```python
from build123d import *

# Parameters (mm, degrees)
SKETCH1_W           = 42
SKETCH1_H           = 70
SKETCH1_R           = 11.5
SKETCH1_R_2         = 1.55
BOSS_EXTRUDE1_DEPTH = 6


with BuildPart() as part:
    # Sketch1 → Boss-Extrude1 (new body)
    with BuildSketch(Plane(origin=(0, 0, 0), x_dir=(1, 0, 0), z_dir=(0, 1, 0))):
        Rectangle(SKETCH1_W, SKETCH1_H)
        with Locations((0, 15)):
            Circle(SKETCH1_R, mode=Mode.SUBTRACT)
        with Locations((-15.5, 30.5)):
            Circle(SKETCH1_R_2, mode=Mode.SUBTRACT)
        with Locations((15.5, 30.5)):
            Circle(SKETCH1_R_2, mode=Mode.SUBTRACT)
        with Locations((15.5, -0.5)):
            Circle(SKETCH1_R_2, mode=Mode.SUBTRACT)
        with Locations((-15.5, -0.5)):
            Circle(SKETCH1_R_2, mode=Mode.SUBTRACT)
        with BuildLine():
            Line((-7.49, -31), (-7.49, -19))
            ThreePointArc((-7.49, -19), (-10, -16.49), (-12.51, -19))
            Line((-12.51, -19), (-12.51, -31))
            ThreePointArc((-12.51, -31), (-10, -33.51), (-7.49, -31))
        make_face(mode=Mode.SUBTRACT)
        with BuildLine():
            Line((-2.51, -31), (-2.51, -19))
            ThreePointArc((-2.51, -19), (0, -16.49), (2.51, -19))
            Line((2.51, -19), (2.51, -31))
            ThreePointArc((2.51, -31), (0, -33.51), (-2.51, -31))
        make_face(mode=Mode.SUBTRACT)
        with BuildLine():
            Line((7.49, -31), (7.49, -19))
            ThreePointArc((7.49, -19), (10, -16.49), (12.51, -19))
            Line((12.51, -19), (12.51, -31))
            ThreePointArc((12.51, -31), (10, -33.51), (7.49, -31))
        make_face(mode=Mode.SUBTRACT)
    extrude(amount=BOSS_EXTRUDE1_DEPTH)


solid = part.part
```
Model file for the job. Use its own axes, mm. A direction names the side the tool comes from. Give positions to 0.01 mm unless a question says otherwise; leave off trailing zeros. Write each loop counter-clockwise with the first axis right and the second up, starting at its lowest first coordinate (ties: lowest second). Pieces come first, ordered by that corner, then holes. Notation, with made-up numbers: (-18, 82.25) -> (-4, 82.25) arc R11 cw to (-4, 88.25) -> close; hole circle Ø2 at (40, 41). An arc over 180 degrees is marked (long way). Use CSV: the item, a comma, the result in double quotes. Start each with the question number.
1) Cut at D-D on x = 15.5. List the corners of the cut face in (y, z), plus the area to 3 significant figures.
2) Cut at A-A on z = 24.5. List the corners of the cut face in (x, y), plus the area to 3 significant figures.
3) Cut at B-B on y = 2.75. Count the separate pieces of the cut face and the enclosed holes in it, plus the area to 3 significant figures.
4) Cut at C-C on z = -30.5. List the corners of the cut face in (x, y).
5) Drill centre lines: L1, parallel to Z at x = 15.5, y = 3.95; L2, parallel to X at y = 2.8, z = -30.5; L3, parallel to X at y = 1.55, z = 22.5. Where is each one in solid material? Low to high.
6) Pin check, flat tip, straight feed: P1, Ø20.5, axis at x = 0, z = -15, coming from the +Y side. Stop position of the tip, or through.
7) Tool access for faces 4 (the flat face through (0, 6, 0)), 5 (the flat face through (2.51, 3, 25)): list every direction of +Z, -Z, +X, -X, +Y, -Y with a clear straight run to the whole face (end or side of a thin tool).
8) Two-plate mould, pull along Z, no slides. Class faces 1 (the cylindrical face through (0.06, 2.96, 33.51)), 2 (the cylindrical face through (9.94, 2.96, 16.49)), 3 (the flat face through (21, 3, 0)): released by +Z, released by -Z, zero draft, split by the parting line, or undercut.
Final values:
1,outline,"(0, -35) -> (6, -35) -> (6, -32.05) -> (0, -32.05) -> close; (0, -28.95) -> (6, -28.95) -> (6, -1.05) -> (0, -1.05) -> close; (0, 2.05) -> (6, 2.05) -> (6, 35) -> (0, 35) -> close"
1,area,"383 mm2"
2,outline,"(-21, 0) -> (-12.51, 0) -> (-12.51, 6) -> (-21, 6) -> close; (-7.49, 0) -> (-2.51, 0) -> (-2.51, 6) -> (-7.49, 6) -> close; (2.51, 0) -> (7.49, 0) -> (7.49, 6) -> (2.51, 6) -> close; (12.51, 0) -> (21, 0) -> (21, 6) -> (12.51, 6) -> close"
2,area,"162 mm2"
3,separate pieces,"1"
3,enclosed holes,"8"
3,area,"2,250 mm2"
4,outline,"(-21, 0) -> (-17.05, 0) -> (-17.05, 6) -> (-21, 6) -> close; (-13.95, 0) -> (13.95, 0) -> (13.95, 6) -> (-13.95, 6) -> close; (17.05, 0) -> (21, 0) -> (21, 6) -> (17.05, 6) -> close"
5,L1,"z = -35 to -32.05, -28.95 to -1.05, 2.05 to 35"
5,L2,"x = -21 to -17.05, -13.95 to 13.95, 17.05 to 21"
5,L3,"x = -21 to -12.51, -7.49 to -2.51, 2.51 to 7.49, 12.51 to 21"
6,P1,"passes through"
7,face 4,"+Z, -Z, +X, -X, +Y"
7,face 5,"+Y, -Y"
8,face 1,"undercut"
8,face 2,"undercut"
8,face 3,"zero draft"
